Geometry: see drawing. Coordinates: mm, zero at the bounding-box minimum. A direction names the side the tool comes from. Coordinates: 2 decimals unless noted, no trailing zeros. Order: outer loops, then holes, each group sorted by start corner. A loop starts at its lowest first (then second) coordinate and runs counter-clockwise, first axis right, second up. Notation, with made-up numbers: (-0.5, 75) - (40.5, 75) arc R14 ccw to (40.5, 91) - close; hole circle Ø10 at (-10.75, 41). An arc over 180 degrees is marked (long way). Use a Markdown table: item, result. Add a question column.
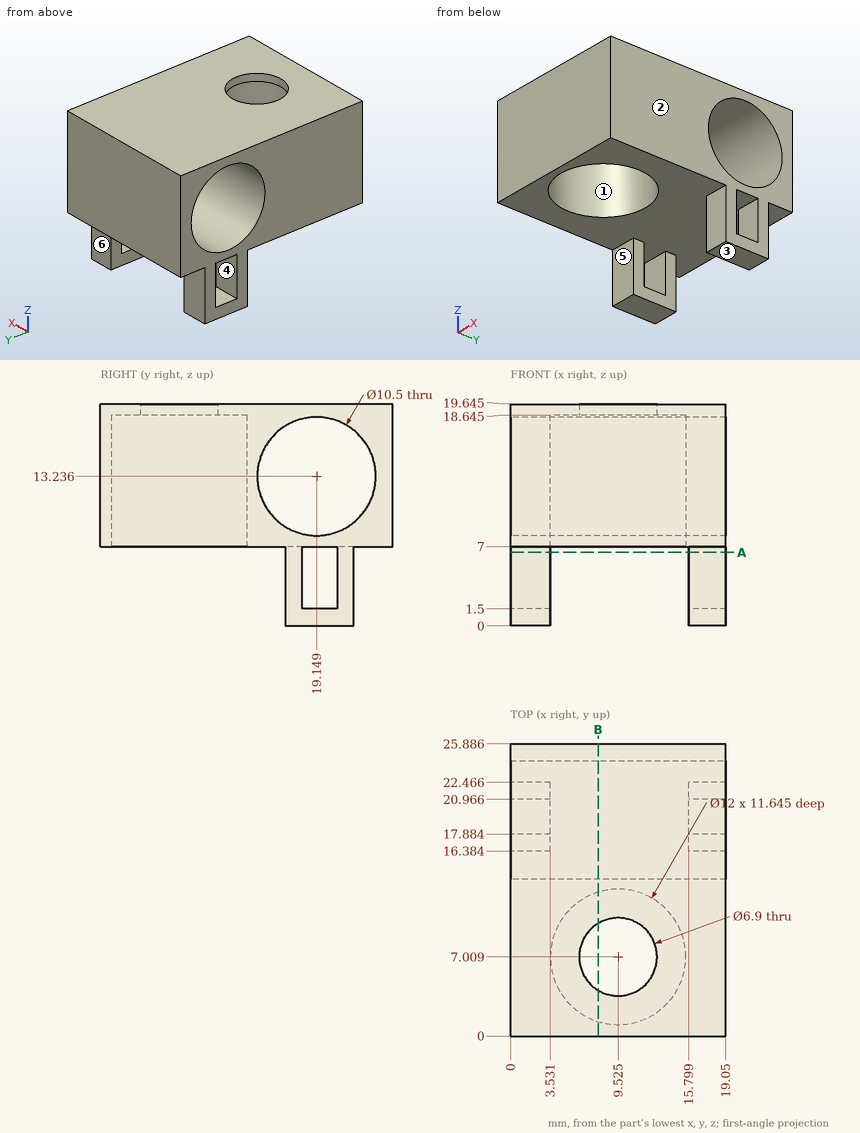
1) Cut plane A-A (z = 6.5). Return the cut outline in (x, y).
2) Material intervals for L1, parallel to Y at x = 17.5, z = 13 (1 decimal); L2, parallel to Y at x = 6.5, z = 14 (1 decimal); L3, parallel to Z at x = 16.25, y = 20.5 (1 decimal), sorted ascending.
3) Cut plane B-B (x = 7.75). State how many separate pieces and enclosed holes the cut face has, and give its area (3 significant figures).
4) Reachability of the marked faces 4, 5 and 6 from +Z, -Z, +X, -X, +Y, -Y: full face, straight path, thin tool, end or side. Return the list, or none.
5) Contact query for flat-ended pins moving along their axis: P1, Ø9.5, axis at x = 10, y = 5.5, coming from the -Z side; P2, Ø3, axis at x = 2, z = 4.5, coming from the +Y side; P3, Ø11, axis at x = 9.52, y = 7.01, coming from the -Z side (1 decimal); P4, Ø4, axis at x = 9.52, y = 7.01, coming from the +Z side. Output: stop coordinate, or through.
6) Pull-direction query (X, two-part tool) for the marked faces 1, 2 and 3; classes: pulls with the +X half, pulls with the -X half, needs draft (parallel to the pull), parting line crosses it, or undercut.
Computed:
| question | item | result |
|---|---|---|
| 1 | outline | (0, 16.38) - (3.53, 16.38) - (3.53, 17.88) - (0, 17.88) - close; (0, 20.97) - (3.53, 20.97) - (3.53, 22.47) - (0, 22.47) - close; (15.8, 16.38) - (19.05, 16.38) - (19.05, 17.88) - (15.8, 17.88) - close; (15.8, 20.97) - (19.05, 20.97) - (19.05, 22.47) - (15.8, 22.47) - close |
| 2 | L1 | y = 0 to 13.9, 24.4 to 25.9 |
| 2 | L2 | y = 0 to 1.8, 12.2 to 14, 24.3 to 25.9 |
| 2 | L3 | z = 0 to 1.5, 7 to 8.2, 18.3 to 19.6 |
| 3 | separate pieces | 2 |
| 3 | enclosed holes | 1 |
| 3 | area | 101 mm2 |
| 4 | face 4 | +X, -X |
| 4 | face 5 | -Z, +X, -X, -Y |
| 4 | face 6 | -Z, +X, -X, +Y |
| 5 | P1 | stops at z = 7 |
| 5 | P2 | stops at y = 22.47 |
| 5 | P3 | stops at z = 18.6 |
| 5 | P4 | passes through |
| 6 | face 1 | undercut |
| 6 | face 2 | pulls with the +X half |
| 6 | face 3 | needs draft |
